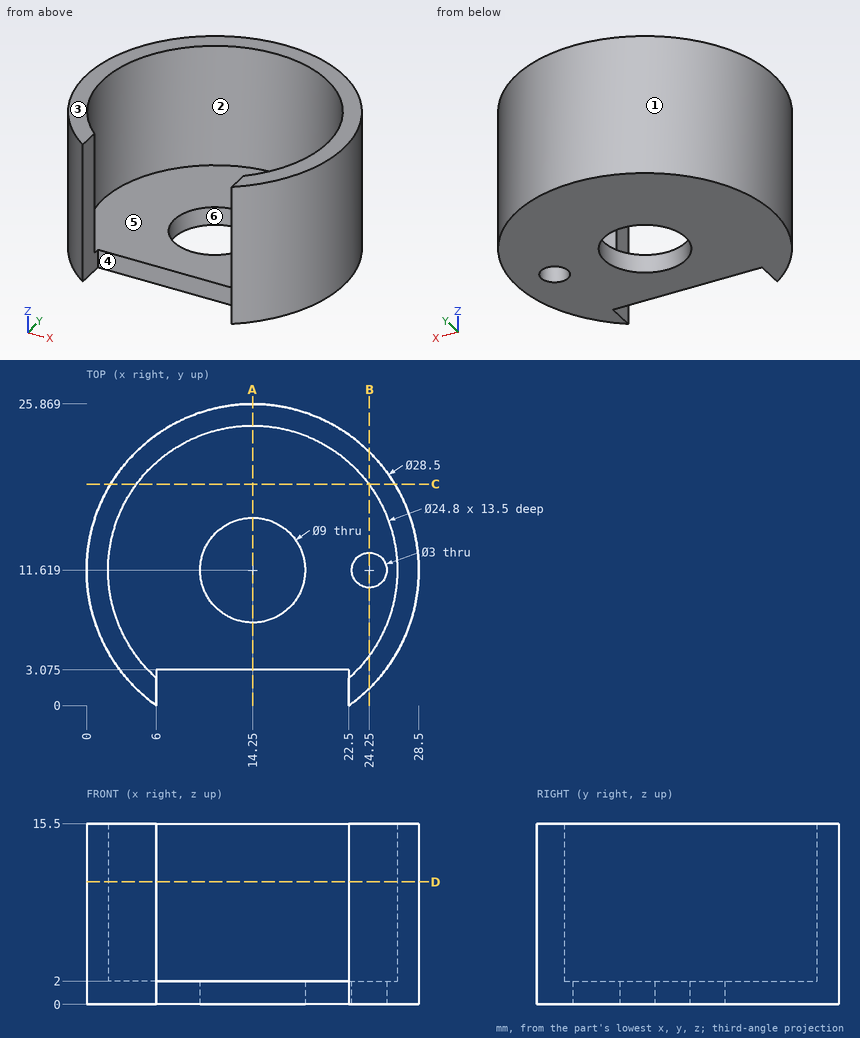
Can you work these out from the drawing? Everything is in mm from the part's minimum corner. A direction names the side the tool comes from. Give positions to 0.01 mm unless a question says otherwise; leave off trailing zeros. Order: outer loops, then holes, each group sorted by start corner. A loop starts at its lowest first (then second) coordinate and runs counter-clockwise, first axis right, second up. Notation, with made-up numbers: M 22.5,49.5 L 56.5,49.5 A28 cw 56.5,68.5 Z; hole C 46,51 d6. An arc over 180 degrees is marked long. Use a Markdown table: item, result. Add a question column.
1. Suppose I cut it at C-C (y = 19). List the corners of the cut face in (x, z) for me.
2. Suppose I cut it at A-A (x = 14.25). List the corners of the cut face in (y, z) for me (3 decimals).
3. On a 3-axis mill with a long thin cutter (end or side, diameter ignored), from which of +Z, -Z, +X, -X, +Y, -Y can I reach the whole of each face in a straight line? I mean the marked faces 5 and 6. Say none if no direction works.
4. For pin 1 Ø2.5 at (y, z) = (1.5, 11) entering from -X; pin 2 Ø1.6 at (x, z) = (16.5, 1) entering from -Y (3 decimals); pin 3 Ø2 at (y, z) = (5, 11.5) entering from +X; pin 4 Ø2.5 at (x, y) = (24.25, 11.62) entering from -Z, each with a flat end and sliding along its axis, tell me the tip position at first contact or that it passes through.
5. If we mould it in two halves opening along X, with no side actions, what happens to the marked faces 1, 2, 3 and 4? For each: +X half, -X half, draft (parallel to the pull), parting line (faces both ways), or undercut.
6. Suppose I cut it at D-D (z = 10.5). List the corners of the cut face in (x, y) for me.
7. Suppose I cut it at B-B (x = 24.25). List the corners of the cut face in (y, z) for me, and give its area (3 significant figures).
8. I need wall thicknesses on probe 1 along Y at (x, z) = (14.25, 1.55) (3 decimals); probe 2 along X at (y, z) = (22, 6); probe 3 along X at (y, z) = (5.25, 8.75). Which ranges of each line are inside material? Lowest first, please. Write a range as from..to.
Results list:
| question | item | result |
|---|---|---|
| 1 | outline | M 2.06,0 L 26.44,0 L 26.44,15.5 L 24.21,15.5 L 24.21,2 L 4.29,2 L 4.29,15.5 L 2.06,15.5 Z |
| 2 | outline | M 3.075,0 L 7.119,0 L 7.119,2 L 3.075,2 Z; M 16.119,0 L 25.869,0 L 25.869,15.5 L 24.019,15.5 L 24.019,2 L 16.119,2 Z |
| 3 | face 5 | +Z |
| 3 | face 6 | +Z, -Z |
| 4 | pin 1 | stops at x = 3.1 |
| 4 | pin 2 | stops at y = 3.075 |
| 4 | pin 3 | stops at x = 27.35 |
| 4 | pin 4 | passes through |
| 5 | face 1 | parting line |
| 5 | face 2 | undercut |
| 5 | face 3 | draft |
| 5 | face 4 | undercut |
| 6 | outline | M 6,0 L 6,2.36 A12.4 cw long 22.5,2.36 L 22.5,0 A14.25 ccw long Z |
| 7 | outline | M 1.47,0 L 10.12,0 L 10.12,2 L 4.29,2 L 4.29,15.5 L 1.47,15.5 Z; M 13.12,0 L 21.77,0 L 21.77,15.5 L 18.95,15.5 L 18.95,2 L 13.12,2 Z |
| 7 | area | 111 mm² |
| 8 | probe 1 | y = 3.075..7.119, 16.119..25.869 |
| 8 | probe 2 | x = 4.49..7.47, 21.03..24.01 |
| 8 | probe 3 | x = 1.5..3.61, 24.89..27 |
